Verification items for the finished model (mm, model axes). A direction names the side the tool comes from. Give positions to 0.01 mm unless a question says otherwise; leave off trailing zeros. Loops run counter-clockwise (first coordinate to the right, second up) from the corner with the lowest first, then second, coordinate; pieces in that order, holes last. Notation, with made-up numbers: (24, 17.25) - (70, 17.25) arc R22 ccw to (70, 26.25) - close; hole circle Ø2 at (7.5, -1.5). An arc over 180 degrees is marked (long way). Answer in a Markdown table with one row per item.
```python
from build123d import *

# Parameters (mm, degrees)
SKETCH_1_R      = 4.25
EXTRUDE_1_DEPTH = 5
FILLET_1_R      = 5
FILLET_2_R      = 15


with BuildPart() as part:
    # Эскиз1 → Бобышка-Вытянуть1 (new body)
    with BuildSketch(Plane.XY):
        with BuildLine():
            Line((-10, -51.794871795), (-10, 108.205128205))
            ThreePointArc((-10, 108.205128205), (-7.902117399, 111.066279057), (-4.542543867, 109.925857514))
            Line((-4.542543867, 109.925857514), (0.279270691, 103.039592664))
            ThreePointArc((0.279270691, 103.039592664), (0.776237817, 100.797918822), (-0.457456133, 98.861407222))
            Line((-0.457456133, 98.861407222), (-2.635311734, 97.336456313))
            ThreePointArc((-2.635311734, 97.336456313), (-4.298968487, 95.353787401), (-4.748403042, 92.804917378))
            Line((-4.748403042, 92.804917378), (6.704486397, -38.102207936))
            ThreePointArc((6.704486397, -38.102207936), (11.513553755, -47.854031847), (21.647406869, -51.794871795))
            Line((21.647406869, -51.794871795), (35, -51.794871795))
            Line((35, -51.794871795), (35, -46.794871795))
            ThreePointArc((35, -46.794871795), (40, -41.794871795), (45, -46.794871795))
            Line((45, -46.794871795), (45, -61.794871795))
            Line((45, -61.794871795), (0, -61.794871795))
            ThreePointArc((0, -61.794871795), (-7.071067812, -58.865939607), (-10, -51.794871795))
        make_face()
        with Locations((0, -51.794871795)):
            Circle(SKETCH_1_R, mode=Mode.SUBTRACT)
    extrude(amount=EXTRUDE_1_DEPTH)

    # Скругление1
    fillet_1_edges = [part.edges().sort_by_distance(p)[0] for p in [
        (35, -51.794871795, 2.5),
    ]]
    fillet(fillet_1_edges, radius=FILLET_1_R - 0.0001)  # a hair under: the kernel refuses the full size

    # Скругление2
    fillet_2_edges = [part.edges().sort_by_distance(p)[0] for p in [
        (45, -61.794871795, 2.5),
    ]]
    fillet(fillet_2_edges, radius=FILLET_2_R - 0.0001)  # a hair under: the kernel refuses the full size


solid = part.part
```
Q1. Draft check along X on faces 4 (the face through (-2.165, 106.531, 2.465)), 5 (the face through (26, -51.795, 2)), 6 (the face through (-10, 27, 2)). Enter one of: +X half, -X half, draft (parallel to the pull), parting line (faces both ways), or undercut.
Completed:
| item | result |
|---|---|
| face 4 | +X half |
| face 5 | undercut |
| face 6 | -X half |
Q2. Go/stop test with a flat-tipped pin: P1, Ø3, axis at x = -2, z = 3.5, coming from the +Y side. Record where the tip stops, or that it passes through.
Completed:
| item | result |
|---|---|
| P1 | y = 108.44 |
Q3. Sectioned sample at B-B (x = 24.5). Record the cut outline in (y, z).
Completed:
| item | result |
|---|---|
| outline | (-61.79, 0) - (-51.79, 0) - (-51.79, 5) - (-61.79, 5) - close |
Q4. Tool access check on faces 1 (the face through (33.574, -50.291, 2.535)), 2 (the face through (3, -1, 0)), 3 (the face through (0.898, 28.268, 2.465)). Record the directions out of +Z, -Z, +X, -X, +Y, -Y that give a thin tool (end or side, any length) a straight path to the whole face; none if there is none.
Completed:
| item | result |
|---|---|
| face 1 | +Z, -Z, +Y |
| face 2 | -Z, +X, -X, +Y, -Y |
| face 3 | +Z, -Z, +X |
Q5. Sectioned sample at C-C (y = 16). Record the cut outline in (x, z).
Completed:
| item | result |
|---|---|
| outline | (-10, 0) - (1.97, 0) - (1.97, 5) - (-10, 5) - close |
Q6. Thickness scan on line 1 (Y direction, x = 24, z = 4.05); line 2 (Y direction, x = 38, z = 2.2); line 3 (X direction, y = -31, z = 4.2). Record the ranges inside material, lowest first.
Completed:
| item | result |
|---|---|
| line 1 | -61.79 to -51.79 |
| line 2 | -59.48 to -42.21 |
| line 3 | -10 to 6.08 |
